Design review of the part shown in the three views and the two pictorial views. Dimensions are in mm from the part's minimum x, y and z. Give positions to 0.01 mm unless a question says otherwise; leave off trailing zeros. Order: outer loops, then holes, each group sorted by start corner. A loop starts at its lowest first (then second) coordinate and runs counter-clockwise, first axis right, second up.
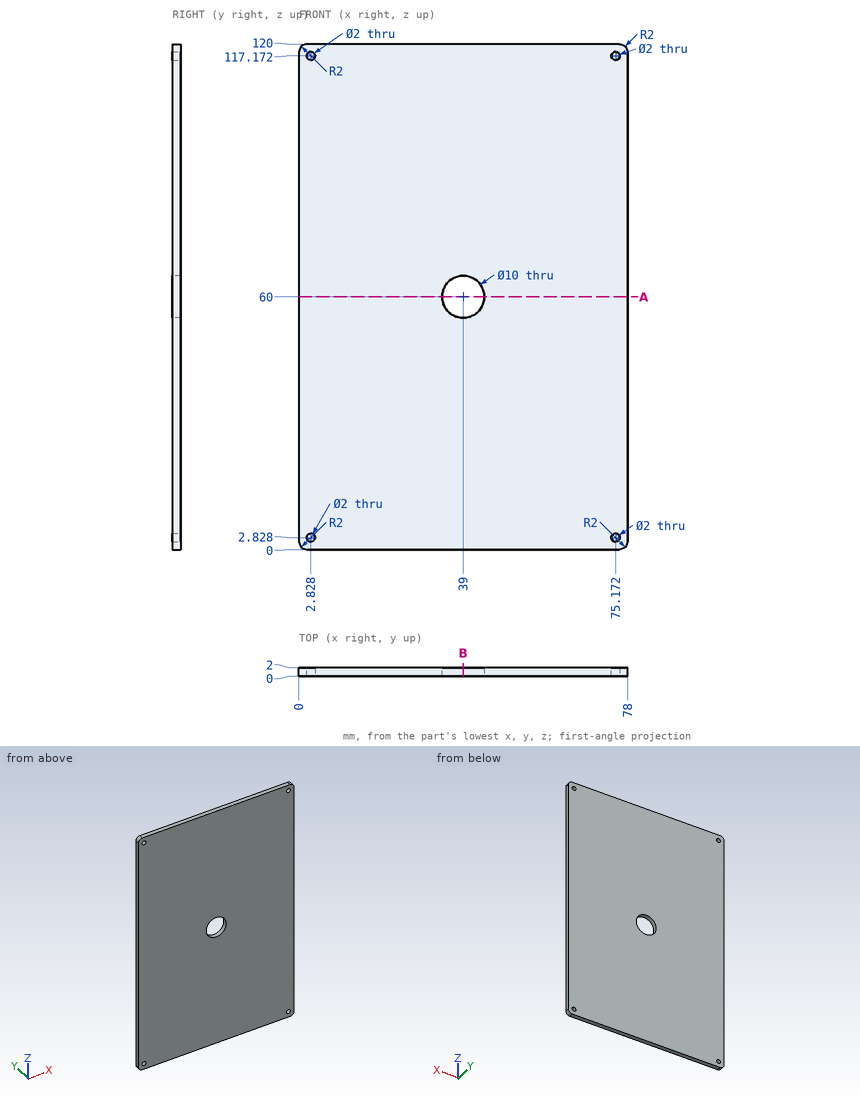
1) We need section B-B on x = 39. Give the boundary of the cut face in (y, z).
Answer sheet:
outline: (0, 0) - (2, 0) - (2, 55) - (0, 55) - close; (0, 65) - (2, 65) - (2, 120) - (0, 120) - close
2) We need section A-A on z = 60. Give the boundary of the cut face in (x, y).
Answer sheet:
outline: (0, 0) - (34, 0) - (34, 2) - (0, 2) - close; (44, 0) - (78, 0) - (78, 2) - (44, 2) - close
3) Clearance check with a flat-ended pin moving along its axis: pin 1 (1.8 mm diameter, centred on x = 2.83, z = 117.17, fed in from -Y). State where the tip first meets the part, or that it passes through.
Answer sheet:
pin 1: passes through
4) To check wall thickness, follow line 1 (Z direction, x = 75, y = 1.5); line 2 (Z direction, x = 39, y = 1); line 3 (X direction, y = 1.15, z = 59.5) (1 decimal). State the ranges of each line that lie inside material, in increasing order.
Answer sheet:
line 1: z = 0 to 1.84, 3.81 to 116.19, 118.16 to 120
line 2: z = 0 to 55, 65 to 120
line 3: x = 0 to 34, 44 to 78
